Verification items for the finished model (mm, model axes). A direction names the side the tool comes from. Give positions to 0.01 mm unless a question says otherwise; leave off trailing zeros. Write each loop counter-clockwise with the first axis right and the second up, starting at its lowest first coordinate (ties: lowest second). Pieces come first, ordered by that corner, then holes. Notation, with made-up numbers: (16, 58.25) -> (66, 58.25) arc R31 cw to (66, 86.25) -> close; hole circle Ø5 at (-38.75, -11). An arc over 180 degrees is marked (long way). Write item = value, one per line.
Autodesk Inventor part; units mm, degrees
ref_plane "YZ Plane" through (0, 0, 0) normal (1, 0, 0) x (0, 1, 0)
ref_plane "XZ Plane" through (0, 0, 0) normal (0, 1, 0) x (-1, 0, 0)
ref_plane "XY Plane" through (0, 0, 0) normal (0, 0, 1) x (1, 0, 0)
sketch "Sketch1" plane through (0, 0, 0) normal (0, 1, 0) x (-1, 0, 0)
  line L0 (0, 0) -> (15, 0)
  line L1 (15, 0) -> (15, -11.5795)
  line L2 (15, -11.5795) -> (5, -8.9)
  line L3 (5, -8.9) -> (5, -21.1)
  line L4 (5, -21.1) -> (15, -18.4205)
  line L5 (15, -18.4205) -> (15, -30)
  line L6 (15, -30) -> (0, -30)
  line L7 (0, -30) -> (0, 0)
  point P0 (5, -15)
  dimension "d0" = 12.2
  dimension "d1" = 30
  dimension "d2" = 15
  dimension "d3" = 10
  dimension "d4" = 30
extrude "Extrusion1" add sketch "Sketch1" along normal blind 60
sketch "Sketch2" plane through (0, 0, 0) normal (0, -1, 0) x (1, 0, 0)
  line L0 (0, -30) -> (-15, -30)
  line L1 (0, 0) -> (0, -30)
  line L2 (-15, 0) -> (0, 0)
  line L3 (-15, -11.5795) -> (-15, 0)
  line L4 (-5, -8.9) -> (-15, -11.5795)
  line L5 (-5, -21.1) -> (-5, -8.9)
  line L6 (-15, -18.4205) -> (-5, -21.1)
  line L7 (-15, -30) -> (-15, -18.4205)
  line L8 (-15, -18.4205) -> (-15, -11.5795)
  circle A0 centre (-10, -15) radius 3
  point P0 (-15, -15)
  point P1 (-10, -19.7603)
  dimension "d9" = 6
extrude "Extrusion2" add sketch "Sketch2" along normal blind 5
properties part number "Laser_Base"
Item 1: Sectioned sample at B-B on y = 2. Record the cut outline in (x, z).
Response values:
outline = (-15, -30) -> (0, -30) -> (0, 0) -> (-15, 0) -> (-15, -11.58) -> (-5, -8.9) -> (-5, -21.1) -> (-15, -18.42) -> close
Item 2: Go/stop test with a flat-tipped pin: P1, Ø1, axis at y = 43, z = -17, coming from the -X side. Record where the tip stops, or that it passes through.
Response values:
P1 = -5
Item 3: Material ranges on line 1 (Z direction, x = -10, y = -2.6); line 2 (Z direction, x = -12.75, y = 2); line 3 (X direction, y = 9, z = -16), recorded low to high.
Response values:
line_1 = -30 to -18, -12 to 0
line_2 = -30 to -19.02, -10.98 to 0
line_3 = -5 to 0
Item 4: Mould release check, pull along Z, two halves, no side actions. Record for faces 3 (the flat face through (-8, 27, -30)), 4 (the flat face through (0, 27, -15)), 5 (the flat face through (-6.7, 0, -14.9)), 6 (the flat face through (-10.07, 29.58, -10.26)): +Z half, -Z half, draft (parallel to the pull), parting line (faces both ways), or undercut.
Response values:
face_3 = -Z half
face_4 = draft
face_5 = undercut
face_6 = undercut
Item 5: Sectioned sample at D-D on z = -10.5. Record the cut outline in (x, y), then the cut area to 3 significant figures.
Response values:
outline = (-15, -5) -> (0, -5) -> (0, 60) -> (-5, 60) -> (-5, 0) -> (-10.97, 0) -> (-10.97, 60) -> (-15, 60) -> close
area = 617 mm^2
Item 6: Sectioned sample at A-A on z = -15. Record the cut outline in (x, y), then the cut area to 3 significant figures.
Response values:
outline = (-15, -5) -> (-13, -5) -> (-13, 0) -> (-15, 0) -> close; (-7, -5) -> (0, -5) -> (0, 60) -> (-5, 60) -> (-5, 0) -> (-7, 0) -> close
area = 345 mm^2
Item 7: Sectioned sample at C-C on x = -10. Record the cut outline in (y, z).
Response values:
outline = (-5, -30) -> (60, -30) -> (60, -19.76) -> (0, -19.76) -> (0, -18) -> (-5, -18) -> close; (-5, -12) -> (0, -12) -> (0, -10.24) -> (60, -10.24) -> (60, 0) -> (-5, 0) -> close
Item 8: Set-up check for faces 1 (the flat face through (-7, 27, 0)), 2 (the flat face through (-9.93, 29.58, -19.78)): record each of +Z, -Z, +X, -X, +Y, -Y from which the full face is reachable in a straight line by a thin tool's end or side.
Response values:
face_1 = +Z, +X, -X, +Y, -Y
face_2 = +Y
